from build123d import *

# Parameters (mm, degrees)
F1_DEPTH = 3.175
F2_R     = 1.1938
F3_DEPTH = 3.175
F4_R     = 2.54
F5_DEPTH = 12.7


with BuildPart() as f1:
    # F0 (on Front) → F1 (new body)
    with BuildSketch(Plane.XZ):
        with BuildLine():
            ThreePointArc((-60.863849, -3.175), (-58.618785, -2.245064), (-57.688849, 0))
            ThreePointArc((-57.688849, 0), (-58.618785, 2.245064), (-60.863849, 3.175))
            ThreePointArc((-60.863849, 3.175), (-64.038849, 0), (-60.863849, -3.175))
        make_face()
        with BuildLine():
            ThreePointArc((-60.863849, 3.175), (-58.618785, 2.245064), (-57.688849, 0))
            ThreePointArc((-57.688849, 0), (-58.618785, -2.245064), (-60.863849, -3.175))
            Line((-60.863849, -3.175), (-22.763849, -3.175))
            ThreePointArc((-22.763849, -3.175), (-25.938849, 0), (-22.763849, 3.175))
            Line((-22.763849, 3.175), (-60.863849, 3.175))
        make_face()
        with BuildLine():
            ThreePointArc((-19.588849, 0), (-20.518785, 2.245064), (-22.763849, 3.175))
            ThreePointArc((-22.763849, 3.175), (-25.938849, 0), (-22.763849, -3.175))
            ThreePointArc((-22.763849, -3.175), (-20.518785, -2.245064), (-19.588849, 0))
        make_face()
    extrude(amount=F1_DEPTH)

    # F2 (on face) → F3 (join)
    with BuildSketch(Plane.XZ.offset(3.175)):
        with Locations((-41.178849, 0)):
            Circle(F2_R)
        with Locations((-59.187449, 0)):
            Circle(F2_R)
    extrude(amount=F3_DEPTH)

    # F4 (on face) → F5 (join)
    with BuildSketch(Plane(origin=(0, 0, 0), x_dir=(-1, 0, 0), z_dir=(0, 1, 0))):
        with Locations((22.763849, 0)):
            Circle(F4_R)
    extrude(amount=F5_DEPTH)


solid = f1.part
Can you work these out from the model? Positions are in its coordinate system, mm. A direction names the side the tool comes from. Round coordinates to 2 decimals unless told otherwise and drop trailing zeros. Write each loop counter-clockwise with the first axis right and the second up, starting at its lowest first coordinate (ties: lowest second). Pieces come first, ordered by that corner, then holes. Notation, with made-up numbers: M 13,82.5 L 46,82.5 A37 ccw 46,118.5 Z; hole C -39.75,65 d1. An arc over 180 degrees is marked long. Use CSV: the item, a comma, the result in double quotes.
(1) We'd pull the mould along X, two halves only. Please class faces 3 (the cylindrical face through (-40.076, -4.74, -0.457)), 4 (the flat face through (-42, -2, 3.175)), 5 (the cylindrical face through (-20.226, 6.261, 0.112)): +X half, -X half, draft (parallel to the pull), parting line (faces both ways), or undercut.
Check values:
face 3,"undercut"
face 4,"draft"
face 5,"parting line"
(2) Imagine slicing it at C-C (y = 8). Write out the boundary of the cut face in (x, z).
Check values:
outline,"C -22.76,0 d5.08"
(3) Imagine slicing it at D-D (x = -41). Write out the boundary of the cut face in (y, z) (3 decimals).
Check values:
outline,"M -6.35,-1.18 L -3.175,-1.18 L -3.175,-3.175 L 0,-3.175 L 0,3.175 L -3.175,3.175 L -3.175,1.18 L -6.35,1.18 Z"
(4) I need wall thicknesses on line 1 along Y through (x, z) = (-47, 0.75) (3 decimals); line 2 along X through (y, z) = (10.25, 2); line 3 along X through (y, z) = (3.75, 1.5). Which ranges of each line are inside material? Lowest first, please.
Check values:
line 1,"-3.175 to 0"
line 2,"-24.33 to -21.2"
line 3,"-24.81 to -20.71"
(5) On a 3-axis mill with a long thin cutter (end or side, diameter ignored), from which of +Z, -Z, +X, -X, +Y, -Y can I reach the whole of each face in a straight line? I mean faces 1 (the flat face through (-42, -2, -3.175)), 2 (the cylindrical face through (-60.38, -4.74, 0.05)). Say none if no direction works.
Check values:
face 1,"-Z, +X, -X, +Y, -Y"
face 2,"-Y"
(6) I'm going to push flat-ended pins straight in: pin 1 (1.9 mm diameter, centred on x = -43.5, z = 1.5, fed in from +Y); pin 2 (1.5 mm diameter, centred on x = -31, z = -2.5, fed in from -Y) (3 decimals). Where does each tip first touch, or does it pass through?
Check values:
pin 1,"y = 0"
pin 2,"y = -3.175"
(7) Imagine slicing it at B-B (z = -1.75). Write out the boundary of the cut face in (x, y) (3 decimals), plus the area to 3 significant figures.
Check values:
outline,"M -63.513,-3.175 L -20.115,-3.175 L -20.115,0 L -20.923,0 L -20.923,12.7 L -24.605,12.7 L -24.605,0 L -63.513,0 Z"
area,"185 mm^2"
(8) Imagine slicing it at A-A (y = -4). Write out the boundary of the cut face in (x, z).
Check values:
outline,"C -59.19,0 d2.39; C -41.18,0 d2.39"
